Geometry: final body of the model. Coordinates: model frame, mm. A direction names the side the tool comes from. Round coordinates to 2 decimals unless told otherwise and drop trailing zeros. Loops run counter-clockwise (first coordinate to the right, second up) from the corner with the lowest first, then second, coordinate; pieces in that order, holes last. Notation, with made-up numbers: (-36.5, 51) - (-9.5, 51) arc R13 cw to (-9.5, 73) - close; hole circle Ø10 at (29, 74). An arc over 180 degrees is marked (long way). Return JSON: item names as keys, results as strings. Group by question number.
1. Section A-A on y = 0. Return loops of the section in (x, z).
2. Draft query along Y for faces 4 (the face through (0, 0, 12)), 5 (the face through (9, 1, 0)), 6 (the face through (20.765, 39.923, 12.325)). Return one class per face: +Y half, -Y half, draft (parallel to the pull), parting line (faces both ways), or undercut.
3. Section B-B on z = 8.75. Return loops of the section in (x, y).
4. Section C-C on x = -7.5. Return loops of the section in (y, z), and give its area (3 significant figures).
5. Section D-D on y = 37.5. Return loops of the section in (x, z), and give its area (3 significant figures).
6. First-contact query: pin 1 Ø2 at (y, z) = (-22, 4.5) entering from -X; pin 2 Ø5.5 at (x, y) = (-29, 29) entering from +Z; pin 3 Ø4.5 at (x, y) = (28.28, -28.28) entering from +Z; pin 4 Ø1.5 at (x, z) = (-9, 9.5) entering from -Y. Flat tips, straight axial feed; report the tip coordinate or a pass-through.
7. Set-up query: faces 1 (the face through (-27, 27, 2)), 2 (the face through (9, 1, 25)), 3 (the face through (-15, 0, 12)). Return all of +Z, -Z, +X, -X, +Y, -Y with unobstructed straight access to the full face (end or side cutting, diameter ignored); none if empty.
8. Material intervals for probe 1 along Y at (x, z) = (-26.5, 8); probe 2 along X at (y, z) = (-15.5, 16); probe 3 along X at (y, z) = (5, 16), sorted ascending.
Autodesk Inventor part; units mm, degrees
ref_plane "YZ Plane" through (0, 0, 0) normal (1, 0, 0) x (0, 1, 0)
ref_plane "XZ Plane" through (0, 0, 0) normal (0, 1, 0) x (-1, 0, 0)
ref_plane "XY Plane" through (0, 0, 0) normal (0, 0, 1) x (1, 0, 0)
sketch "Sketch1" plane through (0, 0, 0) normal (0, 0, 1) x (1, 0, 0)
  circle A0 centre (0, 0) radius 45
  line L0 (-7.5, 25) -> (-7.5, 25)
  line L1 (-15, 17.5) -> (-15, -17.5)
  line L2 (-7.5, -25) -> (-7.5, -25)
  line L3 (0, -17.5) -> (0, 17.5)
  arc A1 (-7.5, 25) -> (-15, 17.5) centre (-7.5, 17.5) ccw
  arc A2 (-15, -17.5) -> (-7.5, -25) centre (-7.5, -17.5) ccw
  arc A3 (-7.5, -25) -> (0, -17.5) centre (-7.5, -17.5) ccw
  arc A4 (0, 17.5) -> (-7.5, 25) centre (-7.5, 17.5) ccw
  point P0 (-15, -25)
  point P1 (-15, 25)
  point P2 (0, -25)
  dimension "d0" = 90
  dimension "d1" = 15
  dimension "d2" = 50
  dimension "d3" = 7.5
  dimension "d4" = 25
  dimension "d5" = 0
extrude "Extrusion1" add sketch "Sketch1" along normal blind 25
sketch "Sketch2" plane through (0, 0, 25) normal (0, 0, 1) x (1, 0, 0)
  line L0 (0, 0) -> (-28.2843, 28.2843)
  line L1 (0, 0) -> (40, 0) construction
  circle A0 centre (-28.2843, 28.2843) radius 2.5
  dimension "d8" = 40
  dimension "d9" = 135
  dimension "d10" = 5
extrude "Extrusion2" cut sketch "Sketch2" against normal blind 23
pattern_circular "Circular Pattern1" count 4 over 360 about axis through (0, 0, 0) along (0, 0, 1) of "Extrusion2"
sketch "Sketch3" plane through (-28.2843, 28.2843, 2) normal (0, 0, 1) x (1, 0, 0)
  circle A0 centre (0, 0) radius 1.25
  point P0 (28.2843, -28.2843)
  dimension "d16" = 2.5
extrude "Extrusion3" cut sketch "Sketch3" against normal blind 3
pattern_circular "Circular Pattern2" count 4 over 360 about axis through (0, 0, 0) along (0, 0, 1) of "Extrusion3"
properties part number "Arm Plate"
Taken from the geometry:
{
 "1": {"outline": "(-45, 0) - (-15, 0) - (-15, 25) - (-45, 25) - close; (0, 0) - (45, 0) - (45, 25) - (0, 25) - close"},
 "2": {"face 4": "undercut", "face 5": "draft", "face 6": "parting line"},
 "3": {"outline": "circle Ø90 at (0, 0); hole circle Ø5 at (-28.28, -28.28); hole circle Ø5 at (-28.28, 28.28); hole (-15, -17.5) arc R7.5 ccw to (0, -17.5) - (0, 17.5) arc R7.5 ccw to (-15, 17.5) - close; hole circle Ø5 at (28.28, -28.28); hole circle Ø5 at (28.28, 28.28)"},
 "4": {"outline": "(-44.37, 0) - (-25, 0) - (-25, 25) - (-44.37, 25) - close; (25, 0) - (44.37, 0) - (44.37, 25) - (25, 25) - close", "area": "969 mm2"},
 "5": {"outline": "(-24.87, 0) - (24.87, 0) - (24.87, 25) - (-24.87, 25) - close", "area": "1,240 mm2"},
 "6": {"pin 1": "x = -39.8", "pin 2": "z = 25", "pin 3": "z = 2", "pin 4": "y = -44.24"},
 "7": {"face 1": "+Z", "face 2": "+Z, +X, -X, +Y, -Y", "face 3": "+Z, -Z"},
 "8": {"probe 1": "-36.37 to -30.04, -26.53 to 26.53, 30.04 to 36.37", "probe 2": "-42.25 to -15, 0 to 42.25", "probe 3": "-44.72 to -15, 0 to 44.72"}
}
